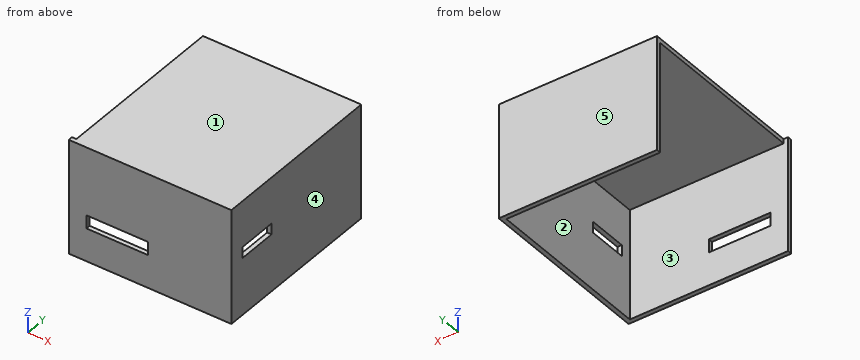
```python
from build123d import *

# Parameters (mm, degrees)
SKIZZE1_W                       = 70
SKIZZE1_H                       = 77
AUFSATZ_LINEAR_AUSTRAGEN1_DEPTH = 2
SKIZZE2_W                       = 52
SKIZZE2_H                       = 77
SKIZZE2_W_2                     = 5
SKIZZE2_H_2                     = 18
AUFSATZ_LINEAR_AUSTRAGEN2_DEPTH = 2
SKIZZE3_W                       = 74
SKIZZE3_H                       = 52
SKIZZE3_W_2                     = 28
SKIZZE3_H_2                     = 6
AUFSATZ_LINEAR_AUSTRAGEN3_DEPTH = 2
SKIZZE9_W                       = 72
SKIZZE9_H                       = 52
AUFSATZ_LINEAR_AUSTRAGEN7_DEPTH = 2


with BuildPart() as part:
    # Skizze1 → Aufsatz-Linear austragen1 (new body)
    with BuildSketch(Plane.XY):
        with Locations((-44.446663724, -34.290378007)):
            Rectangle(SKIZZE1_W, SKIZZE1_H)
    extrude(amount=AUFSATZ_LINEAR_AUSTRAGEN1_DEPTH)

    # Skizze2 → Aufsatz-Linear austragen2 (add)
    with BuildSketch(Plane(origin=(-9.446663724, 0, 0), x_dir=(0, 0, -1), z_dir=(1, 0, 0))):
        with Locations((24, -34.290378007)):
            Rectangle(SKIZZE2_W, SKIZZE2_H)
        with Locations((21.5, -58.790378007)):
            Rectangle(SKIZZE2_W_2, SKIZZE2_H_2, mode=Mode.SUBTRACT)
    extrude(amount=AUFSATZ_LINEAR_AUSTRAGEN2_DEPTH)

    # Skizze3 → Aufsatz-Linear austragen3 (add)
    with BuildSketch(Plane.XZ.offset(72.790378007)):
        with Locations((-44.446663724, -24)):
            Rectangle(SKIZZE3_W, SKIZZE3_H)
        with Locations((-59.397812879, -32)):
            Rectangle(SKIZZE3_W_2, SKIZZE3_H_2, mode=Mode.SUBTRACT)
    extrude(amount=AUFSATZ_LINEAR_AUSTRAGEN3_DEPTH)

    # Skizze9 → Aufsatz-Linear austragen7 (add)
    with BuildSketch(Plane(origin=(0, 4.209621993, 0), x_dir=(1, 0, 0), z_dir=(0, 1, 0))):
        with Locations((-43.446663724, 24)):
            Rectangle(SKIZZE9_W, SKIZZE9_H)
    extrude(amount=AUFSATZ_LINEAR_AUSTRAGEN7_DEPTH)


solid = part.part
```
For this review, take the finished solid that the model builds, in its own axes (mm). Face numbers are marked on the shaded views. A direction names the side the tool comes from. Coordinates: 2 decimals unless noted, no trailing zeros. Loops run counter-clockwise (first coordinate to the right, second up) from the corner with the lowest first, then second, coordinate; pieces in that order, holes last. Notation, with made-up numbers: (47, 12.25) - (54, 12.25) arc R18 ccw to (54, 40.25) - close; hole circle Ø6 at (73.5, 78). An arc over 180 degrees is marked (long way). Use one line per item in the form item = value. Start each with the question number.
1) For pin 1 (1 mm diameter, centred on x = -69.5, y = -64.5, fed in from -Z); pin 2 (25 mm diameter, centred on y = -52.5, z = -17.5, fed in from -X), all flat-tipped, find the tip position at first contact; note any pin that passes through.
2) Take a section at C-C (z = -11.5). State the section outline as (x, y) points, plus the area to 3 significant figures.
3) Draft analysis for pull direction Y (two halves, no side actions). For the marked faces 3, 4 and 5, state which applies: released by +Y, released by -Y, zero draft, split by the parting line, or undercut.
4) For the marked faces 1 and 2, list the 3-axis set-ups (+Z, -Z, +X, -X, +Y, -Y) from which the entire face can be reached by the end or side of a thin tool; tool diameter is ignored.
5) Take a section at B-B (y = -65.5). State the section outline as (x, z) points, plus the area to 3 significant figures.
6) To check wall thickness, follow probe 1 along Y at (x, z) = (-37.5, -30); probe 2 along X at (y, z) = (-50.5, -41.5); probe 3 along Z at (x, y) = (-28.5, -58). State the ranges of each line that lie inside material, in increasing order. Write a range as from..to.
7) Take a section at A-A (x = -61.5). State the section outline as (y, z) points.
8) Take a section at D-D (x = -21). State the section outline as (y, z) points, plus the area to 3 significant figures.
From the geometry:
q1.pin_1 = 0
q1.pin_2 = -9.45
q2.outline = (-81.45, -74.79) - (-7.45, -74.79) - (-7.45, 6.21) - (-79.45, 6.21) - (-79.45, 4.21) - (-9.45, 4.21) - (-9.45, -72.79) - (-81.45, -72.79) - close
q2.area = 446 mm2
q3.face_3 = undercut
q3.face_4 = zero draft
q3.face_5 = released by +Y
q4.face_1 = +Z, +X, -X, +Y, -Y
q4.face_2 = -Z, -X
q5.outline = (-79.45, 0) - (-9.45, 0) - (-9.45, -19) - (-7.45, -19) - (-7.45, 2) - (-79.45, 2) - close; (-9.45, -50) - (-7.45, -50) - (-7.45, -24) - (-9.45, -24) - close
q5.area = 234 mm2
q6.probe_1 = -74.79..-72.79, 4.21..6.21
q6.probe_2 = -9.45..-7.45
q6.probe_3 = 0..2
q7.outline = (-74.79, -50) - (-72.79, -50) - (-72.79, -35) - (-74.79, -35) - close; (-74.79, -29) - (-72.79, -29) - (-72.79, 0) - (4.21, 0) - (4.21, -50) - (6.21, -50) - (6.21, 2) - (-74.79, 2) - close
q8.outline = (-74.79, -50) - (-72.79, -50) - (-72.79, 0) - (4.21, 0) - (4.21, -50) - (6.21, -50) - (6.21, 2) - (-74.79, 2) - close
q8.area = 362 mm2
